The figure shows three views and two pictorial views of one solid part (mm, origin at its lowest corner). Answer the questions. A direction names the side the tool comes from. Give positions to 0.01 mm unless a question says otherwise; leave off trailing zeros. Write each loop counter-clockwise with the first axis right and the second up, starting at its lowest first coordinate (ties: lowest second). Pieces come first, ordered by that corner, then holes. Notation, with made-up numbers: (14, 21.5) - (55, 21.5) arc R18 ccw to (55, 41.5) - close; hole circle Ø11 at (45.25, 89.5). An arc over 180 degrees is marked (long way). Write each question's results on one line, items separated by ' | '. Start each with the question number.
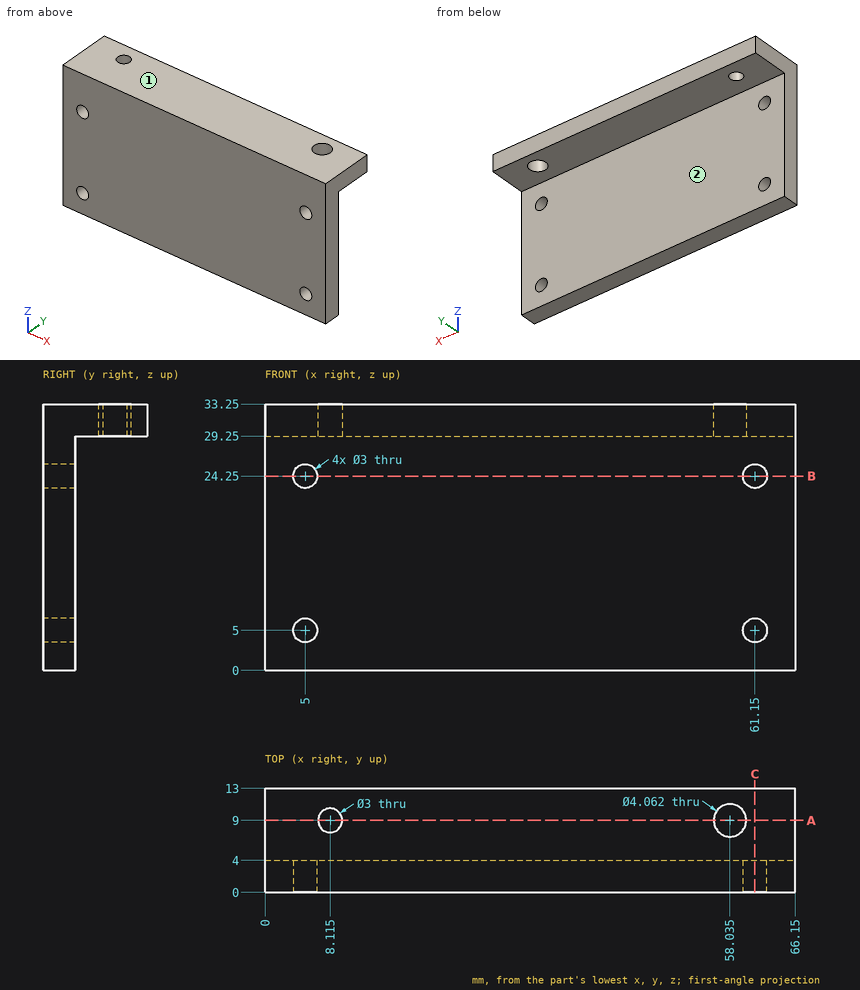
Q1. A tool of negligible diameter and unlimited length cuts with its end or side. For the marked faces 1 and 2, from which of +Z, -Z, +X, -X, +Y, -Y can it reach the whole face along a straight path? Write none if from no direction.
Q2. Consider L1, parallel to Z at x = 61.15, y = 2.45; L2, parallel to X at y = 2.85, z = 5; L3, parallel to X at y = 8, z = 30. Determine where each line is inside the solid, lowest interval first.
Q3. A cutting plane is placed at C-C, the plane x = 61.15. Write down the section's boundary in (y, z), and give its area (3 significant figures).
Q4. A cutting plane is placed at A-A, the plane y = 9. Give the number of separate pieces and of enclosed holes in the cut face, and give its area (3 significant figures).
Q5. A cutting plane is placed at B-B, the plane z = 24.25. Write down the section's boundary in (x, y), and give its area (3 significant figures).
Q6. Given pin 1 (3 mm diameter, centred on x = 56, y = 11.5, fed in from -Z); pin 2 (6 mm diameter, centred on x = 59, z = 24, fed in from +Y), each flat-ended and moving along its own axis, determine where each tip first touches the part or whether it passes through.
Result:
1) face 1: +Z, +X, -X, +Y, -Y | face 2: -Z, +X, -X, +Y
2) L1: z = 0 to 3.5, 6.5 to 22.75, 25.75 to 33.25 | L2: x = 0 to 3.5, 6.5 to 59.65, 62.65 to 66.15 | L3: x = 0 to 7, 9.23 to 56.27, 59.8 to 66.15
3) outline: (0, 0) - (4, 0) - (4, 3.5) - (0, 3.5) - close; (0, 6.5) - (4, 6.5) - (4, 22.75) - (0, 22.75) - close; (0, 25.75) - (4, 25.75) - (4, 29.25) - (13, 29.25) - (13, 33.25) - (0, 33.25) - close | area: 145 mm2
4) separate pieces: 3 | enclosed holes: 0 | area: 236 mm2
5) outline: (0, 0) - (3.5, 0) - (3.5, 4) - (0, 4) - close; (6.5, 0) - (59.65, 0) - (59.65, 4) - (6.5, 4) - close; (62.65, 0) - (66.15, 0) - (66.15, 4) - (62.65, 4) - close | area: 241 mm2
6) pin 1: stops at z = 29.25 | pin 2: stops at y = 4
